Check sheet for the modelled part. Datum: model origin and axes. Units: mm. A direction names the side the tool comes from. Coordinates: 2 decimals unless noted, no trailing zeros. Loops run counter-clockwise (first coordinate to the right, second up) from the corner with the lowest first, then second, coordinate; pieces in that order, holes last. Notation, with made-up numbers: (-20.5, 37.25) -> (-7.5, 37.25) arc R16 ccw to (-7.5, 57.25) -> close; hole circle Ø6 at (-18, 71.25). An arc over 180 degrees is marked (long way). Use CSV: the item, a comma, the result in double quotes.
```python
from build123d import *

# Parameters (mm, degrees)
F0_R      = 76.2
F1_DEPTH  = 19.05
F2_R      = 45.974
F3_DEPTH  = 10.16
F8_R      = 73.66
F8_R_2    = 49.149
F9_DEPTH  = 10.16
F10_R     = 76.2
F10_R_2   = 73.66
F11_DEPTH = 3.175
F14_R     = 4.7625
F14_R_2   = 1.5875
F15_DEPTH = 6.35


with BuildPart() as f1:
    # F0 (on Top) → F1 (new body)
    with BuildSketch(Plane.XY):
        Circle(F0_R)
    extrude(amount=F1_DEPTH)

    # F2 (on face) → F3 (cut)
    with BuildSketch(Plane(origin=(0, 0, 0), x_dir=(1, 0, 0), z_dir=(0, 0, -1))):
        Circle(F2_R)
    extrude(amount=-F3_DEPTH, mode=Mode.SUBTRACT)

    # F4 (on Front) → F5 (revolve, cut)
    with BuildSketch(Plane.XZ):
        Polygon((-17.653, 19.05), (-17.653, 16.51), (-20.32, 16.51), (-20.32, 10.16), (0, 10.16), (0, 19.05), align=None)
    revolve(axis=Axis((0, 0, 14.605), (0, 0, -1)), mode=Mode.SUBTRACT)

    # F6 (on Right) → F7 (revolve, cut)
    with BuildSketch(Plane.YZ):
        Polygon((-38.1, 12.8778), (-25.4, 19.05), (0, 19.05), (0, 29.321771), (-86.354569, 29.321771), (-86.354569, 12.8778), align=None)
    revolve(axis=Axis((0, 0, 24.185886), (0, 0, -1)), mode=Mode.SUBTRACT)

    # F8 (on face) → F9 (cut, through all)
    with BuildSketch(Plane(origin=(0, 0, 0), x_dir=(1, 0, 0), z_dir=(0, 0, -1))):
        Circle(F8_R)
        Circle(F8_R_2, mode=Mode.SUBTRACT)
    extrude(amount=-F9_DEPTH, mode=Mode.SUBTRACT)

    # F10 (on face) → F11 (join)
    with BuildSketch(Plane(origin=(0, 0, 0), x_dir=(1, 0, 0), z_dir=(0, 0, -1))):
        Circle(F10_R)
        Circle(F10_R_2, mode=Mode.SUBTRACT)
    extrude(amount=F11_DEPTH)

    # F14 (on face) → F15 (join)
    with BuildSketch(Plane(origin=(0, 0, 10.16), x_dir=(1, 0, 0), z_dir=(0, 0, -1))):
        with Locations((30.48, -18.804579)):
            Circle(F14_R)
        with Locations((30.48, -18.804579)):
            Circle(F14_R_2, mode=Mode.SUBTRACT)
        with Locations((-30.48, -18.804579)):
            Circle(F14_R)
        with Locations((-30.48, -18.804579)):
            Circle(F14_R_2, mode=Mode.SUBTRACT)
    extrude(amount=F15_DEPTH)


solid = f1.part
```
1) Thickness scan on line 1 along Y through (x, z) = (0, 1); line 2 along Y through (x, z) = (0, 12.75). Record the ranges inside material, lowest first. Write a range as from..to.
Answer below:
line 1,"y = -76.2..-73.66, -49.15..-45.97, 45.97..49.15, 73.66..76.2"
line 2,"y = -76.2..-20.32, 20.32..76.2"
2) Access from +Z, -Z, +X, -X, +Y, -Y to the whole of each face (thin tool, end or side, straight path). Record for faces 1 (the cylindrical face through (3.827, -17.233, 17.762)), 2 (the cylindrical face through (2.645, 20.147, 13.291)).
Answer below:
face 1,"+Z, -Z"
face 2,"-Z"
3) Cross-section at D-D on x = 61. Record the boundary of the cut face in (y, z) (3 decimals), and give its area (3 significant figures).
Answer below:
outline,"(-45.667, -3.175) -> (-41.289, -3.175) -> (-41.289, 10.16) -> (41.289, 10.16) -> (41.289, -3.175) -> (45.667, -3.175) -> (45.667, 12.878) -> (-45.667, 12.878) -> close"
area,"365 mm²"
4) Draft check along Y on faces 3 (the conical face through (25.4, 5.64, 18.75)), 4 (the flat face through (-35, -16, 12.878)), 5 (the flat face through (-31, 21, 3.81)). Enter one of: released by +Y, released by -Y, zero draft, split by the parting line, or undercut.
Answer below:
face 3,"split by the parting line"
face 4,"zero draft"
face 5,"undercut"
5) Cross-section at A-A on y = 0. Record the boundary of the cut face in (x, z) (3 decimals), and give its area (3 significant figures).
Answer below:
outline,"(-76.2, -3.175) -> (-73.66, -3.175) -> (-73.66, 10.16) -> (-49.149, 10.16) -> (-49.149, 0) -> (-45.974, 0) -> (-45.974, 10.16) -> (-20.32, 10.16) -> (-20.32, 16.51) -> (-17.653, 16.51) -> (-17.653, 19.05) -> (-25.4, 19.05) -> (-38.1, 12.878) -> (-76.2, 12.878) -> close; (17.653, 16.51) -> (20.32, 16.51) -> (20.32, 10.16) -> (45.974, 10.16) -> (45.974, 0) -> (49.149, 0) -> (49.149, 10.16) -> (73.66, 10.16) -> (73.66, -3.175) -> (76.2, -3.175) -> (76.2, 12.878) -> (38.1, 12.878) -> (25.4, 19.05) -> (17.653, 19.05) -> close"
area,"591 mm²"
6) Go/stop test with flat-tipped pins: pin 1 Ø1.6 at (x, y) = (31, 18) entering from -Z; pin 2 Ø5 at (x, z) = (-37, 14.5) entering from -Y; pin 3 Ø8 at (x, z) = (10.5, 14) entering from -Y. Record where each tip stops, or that it passes through.
Answer below:
pin 1,"stops at z = 3.81"
pin 2,"stops at y = -67.64"
pin 3,"stops at y = -75.91"
7) Cross-section at C-C on z = 6.75. Record the boundary of the cut face in (x, y) (1 decimal), and give its area (3 significant figures).
Answer below:
outline,"circle Ø152.4 at (0, 0); circle Ø98.3 at (0, 0); circle Ø9.5 at (-30.5, 18.8); circle Ø9.5 at (30.5, 18.8); hole circle Ø147.3 at (0, 0); hole circle Ø91.9 at (0, 0); hole circle Ø3.2 at (-30.5, 18.8); hole circle Ø3.2 at (30.5, 18.8)"
area,"2,270 mm²"
